Here's how the part is built. I have some questions about the finished solid (model axes, mm). Face numbers are marked on the shaded views. A direction names the side the tool comes from. Give positions to 0.01 mm unless a question says otherwise; leave off trailing zeros. Write each loop counter-clockwise with the first axis right and the second up, starting at its lowest first coordinate (ties: lowest second). Pieces come first, ordered by that corner, then holes. Notation, with made-up numbers: (42, 29) -> (79, 29) arc R26 ccw to (79, 64) -> close; hole circle Ø11 at (8, 18.5). An arc over 180 degrees is marked (long way). Put each result on its own line as item: value. Start each with the question number.
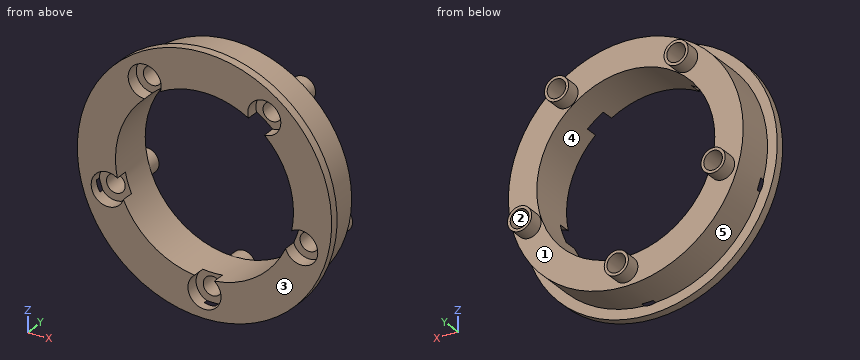
from build123d import *

# Parameters (mm, degrees)
SKETCH3_R           = 27.7
BOSS_EXTRUDE2_DEPTH = 11
SKETCH4_R           = 30
BOSS_EXTRUDE3_DEPTH = 2
SKETCH5_R           = 2.2
CUT_EXTRUDE1_DEPTH  = 44.829214002
SKETCH9_R           = 21
CUT_EXTRUDE5_DEPTH  = 44.829214002
BOSS_EXTRUDE4_START = 3.5
SKETCH10_R          = 2.85
SKETCH10_R_2        = 2.2
BOSS_EXTRUDE4_DEPTH = 3.5
SKETCH15_R          = 3.9
CUT_EXTRUDE6_DEPTH  = 3


with BuildPart() as part:
    # Sketch3 → Boss-Extrude2 (new body)
    with BuildSketch(Plane(origin=(0, 0, 0), x_dir=(1, 0, 0), z_dir=(0, 1, 0))):
        with Locations(Location((0, 0, 0), (0, 0, 270))):
            Circle(SKETCH3_R)
    extrude(amount=BOSS_EXTRUDE2_DEPTH)

    # Sketch4 → Boss-Extrude3 (add)
    with BuildSketch(Plane(origin=(0, 0, 0), x_dir=(1, 0, 0), z_dir=(0, 1, 0))):
        with Locations(Location((0, 0, 0), (0, 0, 270))):
            Circle(SKETCH4_R)
    extrude(amount=BOSS_EXTRUDE3_DEPTH)

    # Sketch5 → Cut-Extrude1 (cut, through all)
    with BuildSketch(Plane(origin=(0, 11, 0), x_dir=(1, 0, 0), z_dir=(0, 1, 0))):
        with Locations(Location((0, 24, 0), (0, 0, 270))):
            Circle(SKETCH5_R)
        with Locations(Location((22.825356391, 7.416407865, 0), (0, 0, 270))):
            Circle(SKETCH5_R)
        with Locations(Location((14.106846055, -19.416407865, 0), (0, 0, 270))):
            Circle(SKETCH5_R)
        with Locations(Location((-14.106846055, -19.416407865, 0), (0, 0, 270))):
            Circle(SKETCH5_R)
        with Locations(Location((-22.825356391, 7.416407865, 0), (0, 0, 270))):
            Circle(SKETCH5_R)
    extrude(amount=-CUT_EXTRUDE1_DEPTH, mode=Mode.SUBTRACT)

    # Sketch9 → Cut-Extrude5 (cut, through all)
    with BuildSketch(Plane(origin=(0, 11, 0), x_dir=(1, 0, 0), z_dir=(0, 1, 0))):
        with Locations(Location((0, 0, 0), (0, 0, 270))):
            Circle(SKETCH9_R)
    extrude(amount=-CUT_EXTRUDE5_DEPTH, mode=Mode.SUBTRACT)

    # Sketch10 → Boss-Extrude4 (add)
    # profile 1 of 5: a face of its own
    with BuildSketch(Plane(origin=(0, 11, 0), x_dir=(1, 0, 0), z_dir=(0, 1, 0)).offset(BOSS_EXTRUDE4_START)):
        with Locations(Location((-22.825356391, 7.416407865, 0), (0, 0, 270))):
            Circle(SKETCH10_R)
        with Locations(Location((-22.825356391, 7.416407865, 0), (0, 0, 270))):
            Circle(SKETCH10_R_2, mode=Mode.SUBTRACT)
    # profile 2 of 5: a face of its own
    with BuildSketch(Plane(origin=(0, 11, 0), x_dir=(1, 0, 0), z_dir=(0, 1, 0)).offset(BOSS_EXTRUDE4_START)):
        with Locations(Location((0, 24, 0), (0, 0, 270))):
            Circle(SKETCH10_R)
        with Locations(Location((0, 24, 0), (0, 0, 270))):
            Circle(SKETCH10_R_2, mode=Mode.SUBTRACT)
    # profile 3 of 5: a face of its own
    with BuildSketch(Plane(origin=(0, 11, 0), x_dir=(1, 0, 0), z_dir=(0, 1, 0)).offset(BOSS_EXTRUDE4_START)):
        with Locations(Location((22.825356391, 7.416407865, 0), (0, 0, 270))):
            Circle(SKETCH10_R)
        with Locations(Location((22.825356391, 7.416407865, 0), (0, 0, 270))):
            Circle(SKETCH10_R_2, mode=Mode.SUBTRACT)
    # profile 4 of 5: a face of its own
    with BuildSketch(Plane(origin=(0, 11, 0), x_dir=(1, 0, 0), z_dir=(0, 1, 0)).offset(BOSS_EXTRUDE4_START)):
        with Locations(Location((14.106846055, -19.416407865, 0), (0, 0, 270))):
            Circle(SKETCH10_R)
        with Locations(Location((14.106846055, -19.416407865, 0), (0, 0, 270))):
            Circle(SKETCH10_R_2, mode=Mode.SUBTRACT)
    # profile 5 of 5: a face of its own
    with BuildSketch(Plane(origin=(0, 11, 0), x_dir=(1, 0, 0), z_dir=(0, 1, 0)).offset(BOSS_EXTRUDE4_START)):
        with Locations(Location((-14.106846055, -19.416407865, 0), (0, 0, 270))):
            Circle(SKETCH10_R)
        with Locations(Location((-14.106846055, -19.416407865, 0), (0, 0, 270))):
            Circle(SKETCH10_R_2, mode=Mode.SUBTRACT)
    extrude(amount=-BOSS_EXTRUDE4_DEPTH)

    # Sketch15 → Cut-Extrude6 (cut)
    with BuildSketch(Plane.XZ):
        with Locations((-14.106846055, 19.416407865)):
            Circle(SKETCH15_R)
        with Locations((14.106846055, 19.416407865)):
            Circle(SKETCH15_R)
        with Locations((22.825356391, -7.416407865)):
            Circle(SKETCH15_R)
        with Locations((0, -24)):
            Circle(SKETCH15_R)
        with Locations((-22.825356391, -7.416407865)):
            Circle(SKETCH15_R)
    extrude(amount=-CUT_EXTRUDE6_DEPTH, mode=Mode.SUBTRACT)


solid = part.part
1) I want a section at B-B, the plane y = 13. State how many separate pieces and enclosed holes the cut face has, and give its area (3 significant figures).
2) Which directions (+Z, -Z, +X, -X, +Y, -Y) give clear straight access to the entire face, cutting with the end or side of a thin tool? Please do the marked faces 1 and 2.
3) I need wall thicknesses on probe 1 along Z at (x, y) = (-16, 9); probe 2 along Z at (x, y) = (-15, 5); probe 3 along X at (y, z) = (13.25, -9). Which ranges of each line are inside material? Lowest first, please.
4) I want a section at C-C, the plane x = 9. Write out the boundary of the cut face in (y, z).
5) I want a section at D-D, the plane x = 0. Write out the boundary of the cut face in (y, z).
6) I'm going to push flat-ended pins straight in: pin 1 Ø4 at (x, z) = (10.5, -20.5) entering from +Y; pin 2 Ø5 at (x, z) = (-22.83, -7.42) entering from -Y; pin 3 Ø6 at (y, z) = (6, -3) entering from +X. Where does each tip first touch, or does it pass through?
7) Thinking about a two-plate mould opening in X: for the marked faces 3, 4 and 5, which applies, released by +X, released by -X, zero draft, split by the parting line, or undercut?
8) I want a section at A-A, the plane z = 0. Write out the boundary of the cut face in (x, y).
Established:
1. separate pieces: 5
1. enclosed holes: 5
1. area: 51.6 mm2
2. face 1: +Y
2. face 2: +Y, -Y
3. probe 1: z = -22.61 to -13.6, 13.6 to 18.3, 20.54 to 22.61
3. probe 2: z = -23.29 to -14.7, 14.7 to 17.41, 21.43 to 23.29
3. probe 3: x = -25.19 to -24.35, -21.3 to -20.46, 20.46 to 21.3, 24.35 to 25.19
4. outline: (0, -28.62) -> (2, -28.62) -> (2, -26.2) -> (11, -26.2) -> (11, -18.97) -> (0, -18.97) -> close; (0, 18.97) -> (11, 18.97) -> (11, 26.2) -> (2, 26.2) -> (2, 28.62) -> (0, 28.62) -> close
5. outline: (0, -30) -> (2, -30) -> (2, -27.9) -> (0, -27.9) -> close; (0, 21) -> (11, 21) -> (11, 27.7) -> (2, 27.7) -> (2, 30) -> (0, 30) -> close; (3, -27.7) -> (11, -27.7) -> (11, -26.85) -> (14.5, -26.85) -> (14.5, -26.2) -> (3, -26.2) -> close; (3, -21.8) -> (14.5, -21.8) -> (14.5, -21.15) -> (11, -21.15) -> (11, -21) -> (3, -21) -> close
6. pin 1: stops at y = 11
6. pin 2: stops at y = 3
6. pin 3: stops at x = 27.7
7. face 3: zero draft
7. face 4: undercut
7. face 5: split by the parting line
8. outline: (-30, 0) -> (-21, 0) -> (-21, 11) -> (-27.7, 11) -> (-27.7, 2) -> (-30, 2) -> close; (21, 0) -> (30, 0) -> (30, 2) -> (27.7, 2) -> (27.7, 11) -> (21, 11) -> close
